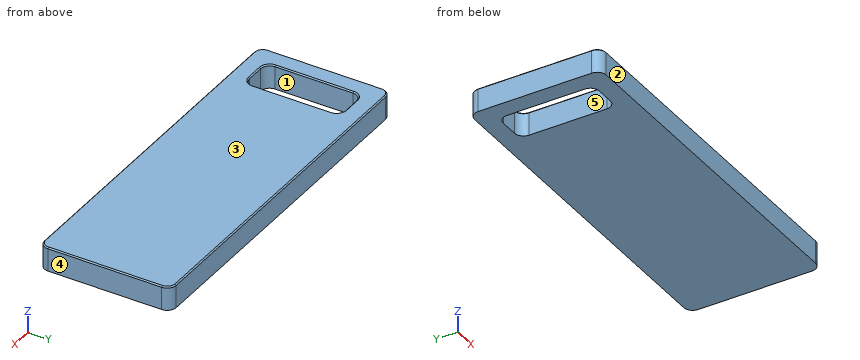
from build123d import *

# Parameters (mm, degrees)
F1_DEPTH = 20
F2_R     = 7.5
F3_SIZE  = 1


with BuildPart() as f1:
    # F0 (on Top) → F1 (new body)
    with BuildSketch(Plane.XY):
        Polygon((0, 55), (0, 0), (300, 0), (300, 110), (0, 110), align=None)
        with BuildLine():
            Line((15, 22.5), (15, 55))
            Line((15, 55), (15, 87.5))
            ThreePointArc((15, 87.5), (17.196699, 92.803301), (22.5, 95))
            Line((22.5, 95), (37.5, 95))
            ThreePointArc((37.5, 95), (42.803301, 92.803301), (45, 87.5))
            Line((45, 87.5), (45, 22.5))
            ThreePointArc((45, 22.5), (42.803301, 17.196699), (37.5, 15))
            Line((37.5, 15), (22.5, 15))
            ThreePointArc((22.5, 15), (17.196699, 17.196699), (15, 22.5))
        make_face(mode=Mode.SUBTRACT)
    extrude(amount=F1_DEPTH)

    # F2
    f2_edges = [f1.edges().sort_by_distance(p)[0] for p in [
        (300, 0, 10),
        (300, 110, 10),
        (0, 0, 10),
        (0, 110, 10),
    ]]
    fillet(f2_edges, radius=F2_R)

    # F3
    f3_edges = [f1.edges().sort_by_distance(p)[0] for p in [
        (0, 55, 20),
        (2.196699, 2.196699, 20),
        (2.196699, 107.803301, 20),
        (150, 0, 20),
        (150, 110, 20),
        (297.803301, 2.196699, 20),
        (297.803301, 107.803301, 20),
        (300, 55, 20),
        (15, 55, 20),
        (17.196699, 92.803301, 20),
        (30, 95, 20),
        (42.803301, 92.803301, 20),
        (45, 55, 20),
        (42.803301, 17.196699, 20),
        (30, 15, 20),
        (17.196699, 17.196699, 20),
    ]]
    chamfer(f3_edges, length=F3_SIZE)


solid = f1.part
Build history of the part. All positions in model axes, mm. Face numbers are marked on the shaded views. A direction names the side the tool comes from. Round coordinates to 2 decimals unless told otherwise and drop trailing zeros. Write each loop counter-clockwise with the first axis right and the second up, starting at its lowest first coordinate (ties: lowest second). Pieces come first, ordered by that corner, then holes. Notation, with made-up numbers: M 22.5,67 L 75.5,67 A18 ccw 75.5,84 Z; hole C 70.5,-35 d2. An arc over 180 degrees is marked long. Answer as a JSON object with one key per item and string values. Group by question number.
(1) Cut at A-A (y = 54). Give the cut face in (x, z).
(2) Which spindle directions (+Z, -Z, +X, -X, +Y, -Y) get a long thin tool onto all of the face, cutting with end or side? Do the marked faces 1 and 2. Say none if no direction does.
(3) Cut at B-B (z = 3.5). Give the cut face in (x, y).
(4) Flat gauge pin, fed straight in: pin 1 (4 mm diameter, centred on x = 263, y = 16.5, fed in from -Z). Where does the tip first touch, or does it go through?
(5) Drill centre lines: L1, parallel to X at y = 28, z = 12; L2, parallel to X at y = 91, z = 16.75; L3, parallel to X at y = 5, z = 11. Where is each one in solid material? Low to high.
(6) Mould opens along X. For the marked faces 3, 4 and 5 say: pulls with the +X half, pulls with the -X half, needs draft (parallel to the pull), parting line crosses it, or undercut.
Responses:
{
 "1": {"outline": "M 0,0 L 15,0 L 15,19 L 14,20 L 1,20 L 0,19 Z; M 45,0 L 300,0 L 300,19 L 299,20 L 46,20 L 45,19 Z"},
 "2": {"face 1": "+Z, -Z", "face 2": "+Z, -Z, +X, -X, -Y"},
 "3": {"outline": "M 0,7.5 A7.5 ccw 7.5,0 L 292.5,0 A7.5 ccw 300,7.5 L 300,102.5 A7.5 ccw 292.5,110 L 7.5,110 A7.5 ccw 0,102.5 Z; hole M 15,22.5 A7.5 ccw 22.5,15 L 37.5,15 A7.5 ccw 45,22.5 L 45,87.5 A7.5 ccw 37.5,95 L 22.5,95 A7.5 ccw 15,87.5 Z"},
 "4": {"pin 1": "stops at z = 0"},
 "5": {"L1": "x = 0 to 15, 45 to 300", "L2": "x = 0 to 15.87, 44.13 to 300", "L3": "x = 0.43 to 299.57"},
 "6": {"face 3": "needs draft", "face 4": "pulls with the +X half", "face 5": "undercut"}
}
